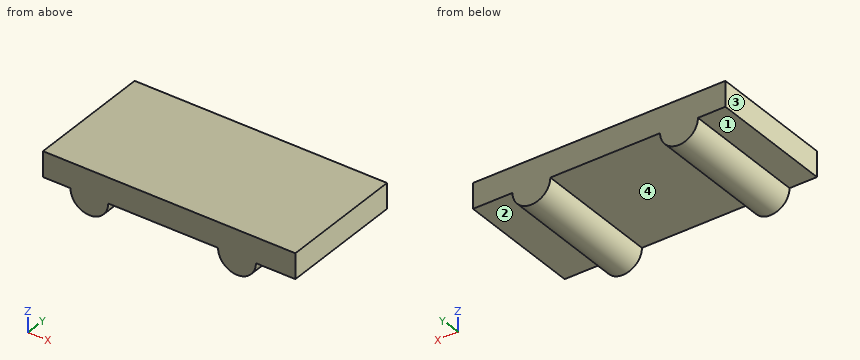
```python
from build123d import *

# Parameters (mm, degrees)
F0_W     = 127
F0_H     = 63.5
F1_DEPTH = 12.7
F4_DEPTH = 63.5


with BuildPart() as f1:
    # F0 (on Top) → F1 (new body)
    with BuildSketch(Plane.XY):
        Rectangle(F0_W, F0_H)
    extrude(amount=F1_DEPTH)

    # F2 (on face) + F3 (on face) → F4 (join)
    with BuildSketch(Plane.XZ.offset(31.75)):
        with BuildLine():
            ThreePointArc((-49.7021888137, 0), (-40.1771888137, -9.525), (-30.6521888137, 0))
            Line((-30.6521888137, 0), (-49.7021888137, 0))
        make_face()
    with BuildSketch(Plane.XZ.offset(31.75)):
        with BuildLine():
            Line((24.5841778814, 0), (43.6341778814, 0))
            ThreePointArc((43.6341778814, 0), (34.1091778814, 9.525), (24.5841778814, 0))
        make_face()
        with BuildLine():
            ThreePointArc((24.5841778814, 0), (34.1091778814, -9.525), (43.6341778814, 0))
            Line((43.6341778814, 0), (24.5841778814, 0))
        make_face()
    extrude(amount=-F4_DEPTH)


solid = f1.part
```
Input: part model. Units: mm. Frame: model coordinates. Face numbers are marked on the shaded views. A direction names the side the tool comes from. Coordinates: 2 decimals unless noted, no trailing zeros. Write each loop counter-clockwise with the first axis right and the second up, starting at its lowest first coordinate (ties: lowest second). Pieces come first, ordered by that corner, then holes. Notation, with made-up numbers: (10, -27.75) -> (14, -27.75) arc R21 cw to (14, -2.75) -> close; hole circle Ø11 at (15.5, 17). An arc over 180 degrees is marked (long way). Write each question's results on one line, items separated by ' | '.
Item 1: Section query C-C on x = 26.5. Return loops of the section in (y, z), plus the area to 3 significant figures.
Conclusion:
outline: (-31.75, -5.73) -> (31.75, -5.73) -> (31.75, 12.7) -> (-31.75, 12.7) -> close | area: 1,170 mm^2
Item 2: Pin query (flat end, axial travel): pin 1 Ø5 at (x, z) = (-28, -3) entering from +Y; pin 2 Ø11 at (x, y) = (-57.5, 2) entering from -Z; pin 3 Ø16 at (x, y) = (49.5, -13) entering from -Z. Return the tip coordinate at first contact, or that it passes through.
Conclusion:
pin 1: passes through | pin 2: stops at z = 0 | pin 3: stops at z = -6.01
Item 3: Section query B-B on x = -55. Return loops of the section in (y, z).
Conclusion:
outline: (-31.75, 0) -> (31.75, 0) -> (31.75, 12.7) -> (-31.75, 12.7) -> close
Item 4: Section query A-A on y = -19. Return loops of the section in (x, z) (3 decimals).
Conclusion:
outline: (-63.5, 0) -> (-49.702, 0) arc R9.525 ccw to (-30.652, 0) -> (24.584, 0) arc R9.525 ccw to (43.634, 0) -> (63.5, 0) -> (63.5, 12.7) -> (-63.5, 12.7) -> close
Item 5: Set-up query: the marked faces 1, 2, 3 and 4. Return all of +Z, -Z, +X, -X, +Y, -Y with unobstructed straight access to the full face (end or side cutting, diameter ignored); none if empty.
Conclusion:
face 1: -Z, -X, +Y, -Y | face 2: -Z, +X, +Y, -Y | face 3: +Z, -Z, -X, +Y, -Y | face 4: -Z, +Y, -Y
Item 6: Material intervals for probe 1 along Z at (x, y) = (-16.5, 9); probe 2 along X at (y, z) = (-8, -4.25); probe 3 along X at (y, z) = (17, -8), sorted ascending.
Conclusion:
probe 1: z = 0 to 12.7 | probe 2: x = -48.7 to -31.65, 25.58 to 42.63 | probe 3: x = -45.35 to -35.01, 28.94 to 39.28
